Input: part model. Units: mm. Frame: model coordinates. Round coordinates to 2 decimals unless told otherwise and drop trailing zeros. Loops run counter-clockwise (first coordinate to the right, second up) from the corner with the lowest first, then second, coordinate; pieces in that order, holes last.
1) Ray query, line 1 along X through (y, z) = (92, 0); line 2 along Z through (x, y) = (-54.5, 67); line 3 along X through (y, z) = (94.5, 25). Return the intervals inside material, ascending.
2) Section B-B, the plane z = -11.5. Return loops of the section in (x, y).
3) Section C-C, the plane y = 52. Return loops of the section in (x, z), and give its area (3 significant figures).
4) Section A-A, the plane x = 51.5. Return loops of the section in (y, z), and give its area (3 significant figures).
5) First-contact query: pin 1 (1 mm diameter, centred on y = 66.5, z = 36.5, fed in from +X); pin 2 (8 mm diameter, centred on x = -35, z = -46, fed in from -Y); pin 3 (3 mm diameter, centred on y = 98.5, z = 21.5, fed in from +X); pin 4 (6 mm diameter, centred on y = 128, z = 26.5, fed in from -X). Flat tips, straight axial feed; report the tip coordinate or a pass-through.
from build123d import *

# Parameters (mm, degrees)
SKETCH1_R           = 63
SKETCH1_R_2         = 61.98
BOSS_EXTRUDE1_DEPTH = 158.49


with BuildPart() as part:
    # Sketch1 → Boss-Extrude1 (new body)
    # profile 1 of 3: a face of its own
    with BuildSketch(Plane(origin=(0, 0, 0), x_dir=(1, 0, 0), z_dir=(0, 1, 0))):
        with BuildLine():
            Line((0, 64.02), (0, 63))
            ThreePointArc((0, 63), (1.984924974, 62.968722973), (3.967879074, 62.874922947))
            Line((3.967879074, 62.874922947), (4.032120926, 63.89289789))
            ThreePointArc((4.032120926, 63.89289789), (2.017061855, 63.988216583), (0, 64.02))
        make_face()
    # profile 2 of 3: a face of its own
    with BuildSketch(Plane(origin=(0, 0, 0), x_dir=(1, 0, 0), z_dir=(0, 1, 0))):
        with BuildLine():
            ThreePointArc((-4.852097182, 62.812874102), (-2.427852094, 62.953201143), (0, 63))
            Line((0, 63), (0, 64.02))
            Line((0, 64.02), (-4.852097182, 62.812874102))
        make_face()
    # profile 3 of 3: a face of its own
    with BuildSketch(Plane(origin=(0, 0, 0), x_dir=(1, 0, 0), z_dir=(0, 1, 0))):
        Circle(SKETCH1_R)
        with Locations(Location((0, 0, 0), (0, 0, 270))):
            Circle(SKETCH1_R_2, mode=Mode.SUBTRACT)
    extrude(amount=BOSS_EXTRUDE1_DEPTH)


solid = part.part
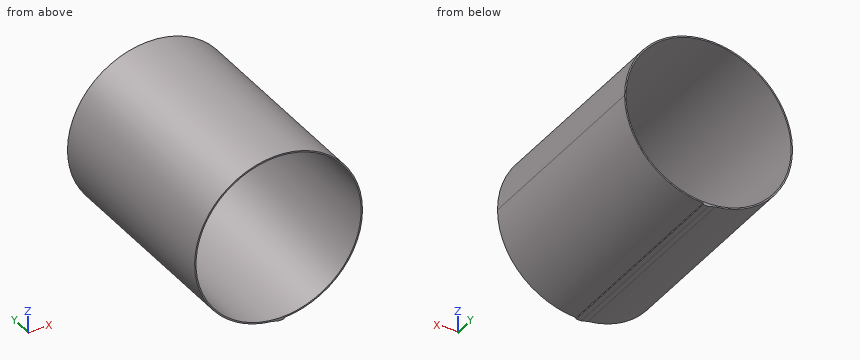
Final values:
1. line 1: x = -63 to -61.98, 61.98 to 63
1. line 2: z = -31.6 to -29.52, 29.52 to 31.6
1. line 3: x = -57.83 to -56.71, 56.71 to 57.83
2. outline: (-61.94, 0) - (-60.9, 0) - (-60.9, 158.49) - (-61.94, 158.49) - close; (60.9, 0) - (61.94, 0) - (61.94, 158.49) - (60.9, 158.49) - close
3. outline: (-4.85, -62.81) - (0, -64.02) arc R64.02 ccw to (4.03, -63.89) - (3.97, -62.87) arc R63 ccw (long way) to start; hole circle Ø123.96 at (0, 0)
3. area: 407 mm2
4. outline: (0, -36.29) - (158.49, -36.29) - (158.49, -34.49) - (0, -34.49) - close; (0, 34.49) - (158.49, 34.49) - (158.49, 36.29) - (0, 36.29) - close
4. area: 571 mm2
5. pin 1: stops at x = 51.7
5. pin 2: passes through
5. pin 3: stops at x = 59.74
5. pin 4: stops at x = -58.45
